Drawing for the job (mm, zero at the part's lowest x, y, z). A direction names the side the tool comes from. Coordinates: 2 decimals unless noted, no trailing zeros. Loops run counter-clockwise (first coordinate to the right, second up) from the corner with the lowest first, then second, coordinate; pieces in that order, holes last. Notation, with made-up numbers: (32, -9.75) -> (70, -9.75) arc R21 cw to (70, 7.25) -> close; hole circle Ø2 at (-16, -35.5). An arc over 180 degrees is marked (long way). Write each question's results on one line, items separated by ' | '.
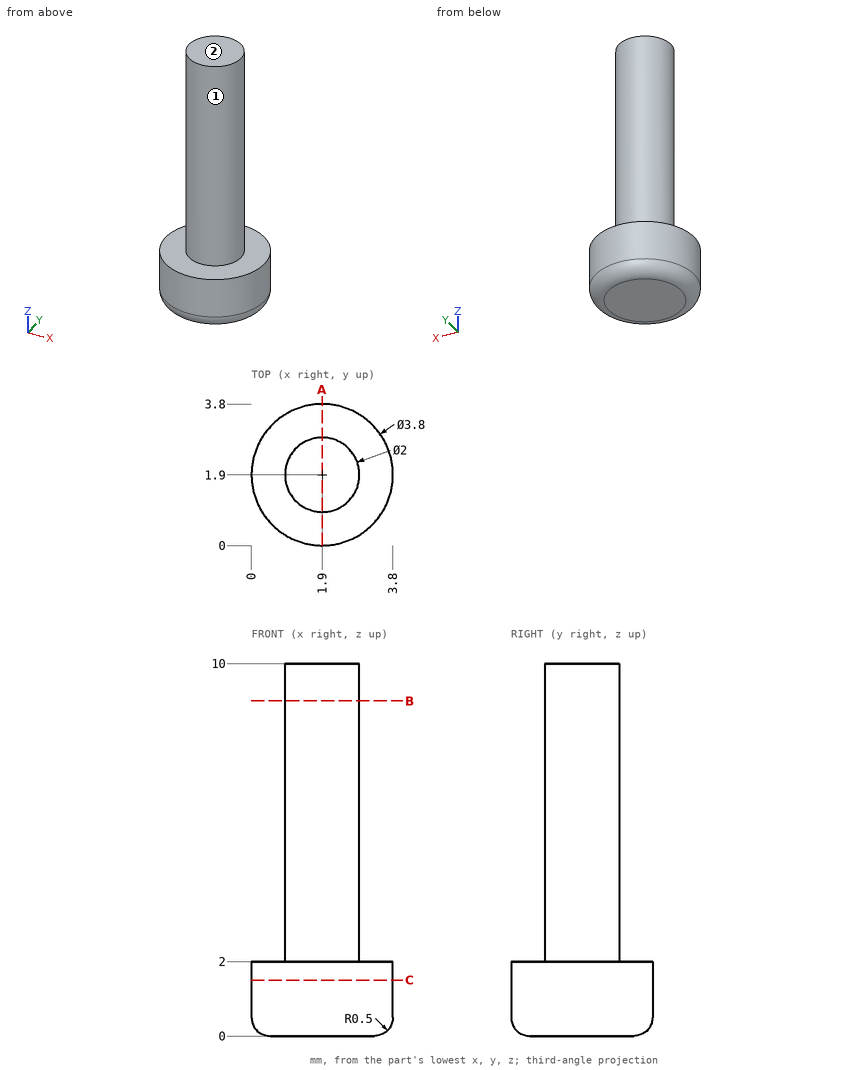
1) Slice it at B-B (z = 9). Write the cut outline in (x, y), then the cut area to 3 significant figures.
Outcome:
outline: circle Ø2 at (1.9, 1.9) | area: 3.14 mm^2
2) Slice it at C-C (z = 1.5). Write the cut outline in (x, y).
Outcome:
outline: circle Ø3.8 at (1.9, 1.9)
3) Which spindle directions (+Z, -Z, +X, -X, +Y, -Y) get a long thin tool onto all of the face, cutting with end or side? Do the marked faces 1 and 2. Say none if no direction does.
Outcome:
face 1: +Z | face 2: +Z, +X, -X, +Y, -Y
4) Slice it at A-A (x = 1.9). Write the cut outline in (y, z).
Outcome:
outline: (0, 0.5) arc R0.5 ccw to (0.5, 0) -> (3.3, 0) arc R0.5 ccw to (3.8, 0.5) -> (3.8, 2) -> (2.9, 2) -> (2.9, 10) -> (0.9, 10) -> (0.9, 2) -> (0, 2) -> close
5) Drill centre lines: L1, parallel to Z at x = 2.45, y = 0.6; L2, parallel to Y at x = 1.85, z = 5.5; L3, parallel to X at y = 0.8, z = 1. Where is each one in solid material? Low to high. Write a range as from..to.
Outcome:
L1: z = 0..2 | L2: y = 0.9..2.9 | L3: x = 0.35..3.45
